Source: CAD feature listing. Evaluate the final solid. Frame: model axes, mm. Round coordinates to 2 decimals unless told otherwise and drop trailing zeros. Write each loop counter-clockwise with the first axis right and the second up, starting at its lowest first coordinate (ties: lowest second). Pieces come first, ordered by that corner, then holes.
from build123d import *

# Parameters (mm, degrees)
SKETCH_1_W          = 70
SKETCH_1_H          = 90
EXTRUDE_1_DEPTH     = 10
SKETCH_2_W          = 15
SKETCH_2_H          = 90
EXTRUDE_2_DEPTH     = 12
EXTRUDE_3_DEPTH     = 3
EXTRUDE_4_DEPTH     = 3
CUT_EXTRUDE_1_REACH = 109.745
SKETCH_7_R          = 6
SKETCH_5_R          = 2.475
CUT_EXTRUDE_2_DEPTH = 22
SKETCH_6_R          = 1.975
CUT_EXTRUDE_4_DEPTH = 10
SKETCH_9_W          = 15
SKETCH_9_H          = 90
CUT_EXTRUDE_5_DEPTH = 1
SKETCH_11_W         = 55
SKETCH_11_H         = 90
CUT_EXTRUDE_6_DEPTH = 116.935326799


with BuildPart() as part:
    # 草图1 → 凸台-拉伸1 (new body)
    with BuildSketch(Plane.XY):
        with Locations((35, 45)):
            Rectangle(SKETCH_1_W, SKETCH_1_H)
    extrude(amount=EXTRUDE_1_DEPTH)

    # 草图2 → 凸台-拉伸2 (add)
    with BuildSketch(Plane.XY.offset(10)):
        with Locations((62.5, 45)):
            Rectangle(SKETCH_2_W, SKETCH_2_H)
    extrude(amount=EXTRUDE_2_DEPTH)

    # 草图3 → 凸台-拉伸3 (add)
    with BuildSketch(Plane(origin=(0, 90, 0), x_dir=(1, 0, 0), z_dir=(0, 1, 0))):
        Polygon((55, -10), (6, -10), (55, -21), align=None)
    extrude(amount=-EXTRUDE_3_DEPTH)

    # 草图4 → 凸台-拉伸4 (add)
    with BuildSketch(Plane.XZ):
        Polygon((55, 21), (6, 10), (55, 10), align=None)
    extrude(amount=-EXTRUDE_4_DEPTH)

    # 草图7 → 切除-拉伸1 (cut, up to next)
    with BuildSketch(Plane.ZY.offset(-55), mode=Mode.PRIVATE) as cut_extrude_1_sk1:
        with Locations((22, 45)):
            Circle(SKETCH_7_R)
    cut_extrude_1_tool1 = extrude(cut_extrude_1_sk1.sketch, amount=-CUT_EXTRUDE_1_REACH, mode=Mode.PRIVATE) & part.part
    add(cut_extrude_1_tool1.solids().sort_by_distance((55, 45, 22))[0], mode=Mode.SUBTRACT)

    # 草图5 → 切除-拉伸2 (cut)
    with BuildSketch(Plane.XY.offset(22)):
        with Locations((62.5, 61)):
            Circle(SKETCH_5_R)
        with Locations((62.5, 29)):
            Circle(SKETCH_5_R)
    extrude(amount=-CUT_EXTRUDE_2_DEPTH, mode=Mode.SUBTRACT)

    # 草图6 → 切除-拉伸4 (cut)
    with BuildSketch(Plane.XY.offset(10)):
        with Locations((3, 29)):
            Circle(SKETCH_6_R)
        with Locations((3, 61)):
            Circle(SKETCH_6_R)
    extrude(amount=-CUT_EXTRUDE_4_DEPTH, mode=Mode.SUBTRACT)

    # 草图9 → 切除-拉伸5 (cut)
    with BuildSketch(Plane.XY.offset(22)):
        with Locations((62.5, 45)):
            Rectangle(SKETCH_9_W, SKETCH_9_H)
    extrude(amount=-CUT_EXTRUDE_5_DEPTH, mode=Mode.SUBTRACT)

    # 草图11 → 切除-拉伸6 (cut, through all)
    with BuildSketch(Plane(origin=(0, 0, 0), x_dir=(-1, 0, 0), z_dir=(0, 0, -1))):
        with Locations((-27.5, 45)):
            Rectangle(SKETCH_11_W, SKETCH_11_H)
    extrude(amount=-CUT_EXTRUDE_6_DEPTH, mode=Mode.SUBTRACT)


solid = part.part
1) Section query B-B on y = 29. Return the cut outline in (x, z) (3 decimals).
Taken from the geometry:
outline: (55, 0) - (60.025, 0) - (60.025, 21) - (55, 21) - close; (64.975, 0) - (70, 0) - (70, 21) - (64.975, 21) - close
2) Section query C-C on z = 19.25. Return the cut outline in (x, y) (3 decimals).
Taken from the geometry:
outline: (55, 0) - (70, 0) - (70, 39.667) - (55, 39.667) - close; (55, 50.333) - (70, 50.333) - (70, 90) - (55, 90) - close; hole circle Ø4.95 at (62.5, 29); hole circle Ø4.95 at (62.5, 61)
3) Section query D-D on z = 8. Return the cut outline in (x, y) (3 decimals), then the cut area to 3 significant figures.
Taken from the geometry:
outline: (55, 0) - (70, 0) - (70, 90) - (55, 90) - close; hole circle Ø4.95 at (62.5, 29); hole circle Ø4.95 at (62.5, 61)
area: 1,310 mm2
4) Material intervals for line 1 (Y direction, x = 62.5, z = 14.25) (3 decimals); line 2 (Y direction, x = 62.5, z = 16.75) (3 decimals); line 3 (X direction, y = 31, z = 17.75), sorted ascending.
Taken from the geometry:
line 1: y = 0 to 26.525, 31.475 to 58.525, 63.475 to 90
line 2: y = 0 to 26.525, 31.475 to 42.095, 47.905 to 58.525, 63.475 to 90
line 3: x = 55 to 61.04, 63.96 to 70
5) Pull-direction query (Y, two-part tool) for faces 1 (the face through (63.831, 31.087, 10.647)), 2 (the face through (62, 0, 11)), 3 (the face through (64.786, 60.052, 10.647)), 4 (the face through (70, 44, 10)); classes: released by +Y, released by -Y, zero draft, split by the parting line, or undercut.
Taken from the geometry:
face 1: undercut
face 2: released by -Y
face 3: undercut
face 4: zero draft
6) Section query A-A on x = 62.5. Return the cut outline in (y, z) (3 decimals).
Taken from the geometry:
outline: (0, 0) - (26.525, 0) - (26.525, 21) - (0, 21) - close; (31.475, 0) - (58.525, 0) - (58.525, 21) - (50.916, 21) arc R6 cw to (39.084, 21) - (31.475, 21) - close; (63.475, 0) - (90, 0) - (90, 21) - (63.475, 21) - close
